Work out the finished part from the listing and answer in its coordinate system (mm). Face numbers are marked on the shaded views. Round coordinates to 2 decimals unless told otherwise and drop trailing zeros. Loops run counter-clockwise (first coordinate to the right, second up) from the corner with the lowest first, then second, coordinate; pieces in that order, holes last.
```python
from build123d import *

# Parameters (mm, degrees)
SKETCH1_R          = 3.175
EXTRUDE1_DEPTH     = 5.4864
CUT_EXTRUDE1_START = -6.349814
SKETCH2_R          = 1.7272
CUT_EXTRUDE1_DEPTH = 12.699628


with BuildPart() as part:
    # Sketch1 → Extrude1 (new body)
    with BuildSketch(Plane.XY):
        Polygon((0, 6.349813731), (-5.4991, 3.174906865), (-5.4991, -3.174906865), (0, -6.349813731), (5.4991, -3.174906865), (5.4991, 3.174906865), align=None)
        Circle(SKETCH1_R, mode=Mode.SUBTRACT)
    extrude(amount=EXTRUDE1_DEPTH)

    # Sketch2 → Cut-Extrude1 (cut)
    with BuildSketch(Plane(origin=(0, 0, 0), x_dir=(0, 0, -1), z_dir=(0, 1, 0)).offset(CUT_EXTRUDE1_START)):
        with Locations((-2.7432, 0)):
            Circle(SKETCH2_R)
    extrude(amount=CUT_EXTRUDE1_DEPTH, mode=Mode.SUBTRACT)


solid = part.part
```
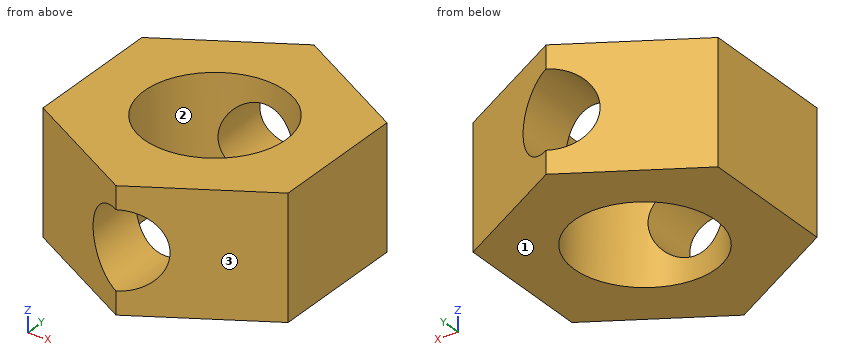
1. Consider probe 1 along Z at (x, y) = (0, 5.2); probe 2 along X at (y, z) = (2, 2.9); probe 3 along X at (y, z) = (1, 3.55). Determine where each line is inside the solid, lowest interval first.
Answer key:
probe 1: z = 0 to 1.02, 4.47 to 5.49
probe 2: x = -5.5 to -2.47, 2.47 to 5.5
probe 3: x = -5.5 to -3.01, 3.01 to 5.5
2. Find section A-A (y = 0). Write down the section's boundary in (x, z) (3 decimals).
Answer key:
outline: (-5.499, 0) - (-3.175, 0) - (-3.175, 5.486) - (-5.499, 5.486) - close; (3.175, 0) - (5.499, 0) - (5.499, 5.486) - (3.175, 5.486) - close
3. Find section C-C (x = 2.25). Write down the section's boundary in (y, z), then the cut area to 3 significant figures.
Answer key:
outline: (-5.05, 0) - (-2.24, 0) - (-2.24, 5.49) - (-5.05, 5.49) - close; (2.24, 0) - (5.05, 0) - (5.05, 5.49) - (2.24, 5.49) - close
area: 30.8 mm2
4. Find section B-B (z = 3.2). Write down the section's boundary in (x, y) (3 decimals), then the cut area to 3 significant figures.
Answer key:
outline: (-5.499, -3.175) - (-1.666, -5.388) - (-1.666, -2.703) arc R3.175 cw to (-1.666, 2.703) - (-1.666, 5.388) - (-5.499, 3.175) - close; (1.666, -5.388) - (5.499, -3.175) - (5.499, 3.175) - (1.666, 5.388) - (1.666, 2.703) arc R3.175 cw to (1.666, -2.703) - close
area: 54.1 mm2
5. Determine the mould class of the marked faces 1, 2 and 3 for opening direction X: +X half, -X half, draft (parallel to the pull), parting line (faces both ways), or undercut.
Answer key:
face 1: draft
face 2: undercut
face 3: +X half
6. Find section D-D (x = -0.5). Write down the section's boundary in (y, z).
Answer key:
outline: (-6.06, 0) - (-3.14, 0) - (-3.14, 1.09) - (-6.06, 1.09) - close; (-6.06, 4.4) - (-3.14, 4.4) - (-3.14, 5.49) - (-6.06, 5.49) - close; (3.14, 0) - (6.06, 0) - (6.06, 1.09) - (3.14, 1.09) - close; (3.14, 4.4) - (6.06, 4.4) - (6.06, 5.49) - (3.14, 5.49) - close
